```python
from build123d import *

# Parameters (mm, degrees)
SKETCH1_R           = 0.375
SKETCH1_R_2         = 0.6
BOSS_EXTRUDE1_DEPTH = 1.25
BOSS_EXTRUDE2_DEPTH = 2.4
BOSS_EXTRUDE3_DEPTH = 4


with BuildPart() as part:
    # Sketch1 → Boss-Extrude1 (new body)
    # profile 1 of 7: a face of its own
    with BuildSketch(Plane(origin=(0, 0, 0), x_dir=(1, 0, 0), z_dir=(0, 1, 0))):
        with BuildLine():
            Line((18.75, 18.75), (13.75, 18.75))
            ThreePointArc((13.75, 18.75), (12.5, 17.5), (11.25, 18.75))
            Line((11.25, 18.75), (-18.75, 18.75))
            Line((-18.75, 18.75), (-18.75, -18.75))
            Line((-18.75, -18.75), (11.25, -18.75))
            ThreePointArc((11.25, -18.75), (12.5, -17.5), (13.75, -18.75))
            Line((13.75, -18.75), (18.75, -18.75))
            Line((18.75, -18.75), (18.75, 18.75))
        make_face()
        with Locations((-18, -18)):
            Circle(SKETCH1_R, mode=Mode.SUBTRACT)
        with BuildLine():
            ThreePointArc((-5.25, 17), (-4.542893219, 16.707106781), (-4.25, 16))
            Line((-4.25, 16), (-4.25, 15.75))
            ThreePointArc((-4.25, 15.75), (-3.957106781, 15.042893219), (-3.25, 14.75))
            Line((-3.25, 14.75), (3.25, 14.75))
            ThreePointArc((3.25, 14.75), (3.957106781, 15.042893219), (4.25, 15.75))
            Line((4.25, 15.75), (4.25, 16))
            ThreePointArc((4.25, 16), (4.542893219, 16.707106781), (5.25, 17))
            Line((5.25, 17), (12, 17))
            ThreePointArc((12, 17), (15.535533906, 15.535533906), (17, 12))
            Line((17, 12), (17, -12))
            ThreePointArc((17, -12), (15.535533906, -15.535533906), (12, -17))
            Line((12, -17), (-12, -17))
            ThreePointArc((-12, -17), (-15.535533906, -15.535533906), (-17, -12))
            Line((-17, -12), (-17, 12))
            ThreePointArc((-17, 12), (-15.535533906, 15.535533906), (-12, 17))
            Line((-12, 17), (-5.25, 17))
        make_face(mode=Mode.SUBTRACT)
        with Locations((16.95, -16.95)):
            Circle(SKETCH1_R_2, mode=Mode.SUBTRACT)
        with Locations((-18, 18)):
            Circle(SKETCH1_R, mode=Mode.SUBTRACT)
        Polygon((16.75, 18.25), (18.25, 18.25), (18.25, 16.75), align=None, mode=Mode.SUBTRACT)
    # profile 2 of 7: a face of its own
    with BuildSketch(Plane(origin=(0, 0, 0), x_dir=(1, 0, 0), z_dir=(0, 1, 0))):
        with BuildLine():
            Line((-4.25, 15.75), (-4.25, 16))
            ThreePointArc((-4.25, 16), (-4.542893219, 16.707106781), (-5.25, 17))
            Line((-5.25, 17), (-12, 17))
            ThreePointArc((-12, 17), (-15.535533906, 15.535533906), (-17, 12))
            Line((-17, 12), (-17, -12))
            ThreePointArc((-17, -12), (-15.535533906, -15.535533906), (-12, -17))
            Line((-12, -17), (12, -17))
            ThreePointArc((12, -17), (15.535533906, -15.535533906), (17, -12))
            Line((17, -12), (17, 12))
            ThreePointArc((17, 12), (15.535533906, 15.535533906), (12, 17))
            Line((12, 17), (5.25, 17))
            ThreePointArc((5.25, 17), (4.542893219, 16.707106781), (4.25, 16))
            Line((4.25, 16), (4.25, 15.75))
            ThreePointArc((4.25, 15.75), (3.957106781, 15.042893219), (3.25, 14.75))
            Line((3.25, 14.75), (12.25, 14.75))
            ThreePointArc((12.25, 14.75), (14.017766953, 14.017766953), (14.75, 12.25))
            Line((14.75, 12.25), (14.75, -12.25))
            ThreePointArc((14.75, -12.25), (14.017766953, -14.017766953), (12.25, -14.75))
            Line((12.25, -14.75), (-12.25, -14.75))
            ThreePointArc((-12.25, -14.75), (-14.017766953, -14.017766953), (-14.75, -12.25))
            Line((-14.75, -12.25), (-14.75, 12.25))
            ThreePointArc((-14.75, 12.25), (-14.017766953, 14.017766953), (-12.25, 14.75))
            Line((-12.25, 14.75), (-3.25, 14.75))
            ThreePointArc((-3.25, 14.75), (-3.957106781, 15.042893219), (-4.25, 15.75))
        make_face()
    # profile 3 of 7: a face of its own
    with BuildSketch(Plane(origin=(0, 0, 0), x_dir=(1, 0, 0), z_dir=(0, 1, 0))):
        with BuildLine():
            Line((12.25, 14.75), (-12.25, 14.75))
            ThreePointArc((-12.25, 14.75), (-14.017766953, 14.017766953), (-14.75, 12.25))
            Line((-14.75, 12.25), (-14.75, -12.25))
            ThreePointArc((-14.75, -12.25), (-14.017766953, -14.017766953), (-12.25, -14.75))
            Line((-12.25, -14.75), (12.25, -14.75))
            ThreePointArc((12.25, -14.75), (14.017766953, -14.017766953), (14.75, -12.25))
            Line((14.75, -12.25), (14.75, 12.25))
            ThreePointArc((14.75, 12.25), (14.017766953, 14.017766953), (12.25, 14.75))
        make_face()
    # profile 4 of 7: a face of its own
    with BuildSketch(Plane(origin=(0, 0, 0), x_dir=(1, 0, 0), z_dir=(0, 1, 0))):
        with Locations((-18, -18)):
            Circle(SKETCH1_R)
    # profile 5 of 7: a face of its own
    with BuildSketch(Plane(origin=(0, 0, 0), x_dir=(1, 0, 0), z_dir=(0, 1, 0))):
        with Locations((16.95, -16.95)):
            Circle(SKETCH1_R_2)
    # profile 6 of 7: a face of its own
    with BuildSketch(Plane(origin=(0, 0, 0), x_dir=(1, 0, 0), z_dir=(0, 1, 0))):
        Polygon((18.25, 18.25), (16.75, 18.25), (18.25, 16.75), align=None)
    # profile 7 of 7: a face of its own
    with BuildSketch(Plane(origin=(0, 0, 0), x_dir=(1, 0, 0), z_dir=(0, 1, 0))):
        with Locations((-18, 18)):
            Circle(SKETCH1_R)
    extrude(amount=BOSS_EXTRUDE1_DEPTH)

    # Sketch1_3 → Boss-Extrude2 (add)
    with BuildSketch(Plane(origin=(0, 0, 0), x_dir=(1, 0, 0), z_dir=(0, 1, 0))):
        with BuildLine():
            Line((-4.25, 15.75), (-4.25, 16))
            ThreePointArc((-4.25, 16), (-4.542893219, 16.707106781), (-5.25, 17))
            Line((-5.25, 17), (-12, 17))
            ThreePointArc((-12, 17), (-15.535533906, 15.535533906), (-17, 12))
            Line((-17, 12), (-17, -12))
            ThreePointArc((-17, -12), (-15.535533906, -15.535533906), (-12, -17))
            Line((-12, -17), (12, -17))
            ThreePointArc((12, -17), (15.535533906, -15.535533906), (17, -12))
            Line((17, -12), (17, 12))
            ThreePointArc((17, 12), (15.535533906, 15.535533906), (12, 17))
            Line((12, 17), (5.25, 17))
            ThreePointArc((5.25, 17), (4.542893219, 16.707106781), (4.25, 16))
            Line((4.25, 16), (4.25, 15.75))
            ThreePointArc((4.25, 15.75), (3.957106781, 15.042893219), (3.25, 14.75))
            Line((3.25, 14.75), (12.25, 14.75))
            ThreePointArc((12.25, 14.75), (14.017766953, 14.017766953), (14.75, 12.25))
            Line((14.75, 12.25), (14.75, -12.25))
            ThreePointArc((14.75, -12.25), (14.017766953, -14.017766953), (12.25, -14.75))
            Line((12.25, -14.75), (-12.25, -14.75))
            ThreePointArc((-12.25, -14.75), (-14.017766953, -14.017766953), (-14.75, -12.25))
            Line((-14.75, -12.25), (-14.75, 12.25))
            ThreePointArc((-14.75, 12.25), (-14.017766953, 14.017766953), (-12.25, 14.75))
            Line((-12.25, 14.75), (-3.25, 14.75))
            ThreePointArc((-3.25, 14.75), (-3.957106781, 15.042893219), (-4.25, 15.75))
        make_face()
        with BuildLine():
            Line((12.25, 14.75), (-12.25, 14.75))
            ThreePointArc((-12.25, 14.75), (-14.017766953, 14.017766953), (-14.75, 12.25))
            Line((-14.75, 12.25), (-14.75, -12.25))
            ThreePointArc((-14.75, -12.25), (-14.017766953, -14.017766953), (-12.25, -14.75))
            Line((-12.25, -14.75), (12.25, -14.75))
            ThreePointArc((12.25, -14.75), (14.017766953, -14.017766953), (14.75, -12.25))
            Line((14.75, -12.25), (14.75, 12.25))
            ThreePointArc((14.75, 12.25), (14.017766953, 14.017766953), (12.25, 14.75))
        make_face()
    extrude(amount=BOSS_EXTRUDE2_DEPTH)

    # Sketch1_4 → Boss-Extrude3 (add)
    with BuildSketch(Plane(origin=(0, 0, 0), x_dir=(1, 0, 0), z_dir=(0, 1, 0))):
        with BuildLine():
            Line((12.25, 14.75), (-12.25, 14.75))
            ThreePointArc((-12.25, 14.75), (-14.017766953, 14.017766953), (-14.75, 12.25))
            Line((-14.75, 12.25), (-14.75, -12.25))
            ThreePointArc((-14.75, -12.25), (-14.017766953, -14.017766953), (-12.25, -14.75))
            Line((-12.25, -14.75), (12.25, -14.75))
            ThreePointArc((12.25, -14.75), (14.017766953, -14.017766953), (14.75, -12.25))
            Line((14.75, -12.25), (14.75, 12.25))
            ThreePointArc((14.75, 12.25), (14.017766953, 14.017766953), (12.25, 14.75))
        make_face()
    extrude(amount=BOSS_EXTRUDE3_DEPTH)


solid = part.part
```
The listing builds one solid part. Answer for the finished solid, in the listing's coordinates (mm). A direction names the side the tool comes from. Round coordinates to 2 decimals unless told otherwise and drop trailing zeros. Loops run counter-clockwise (first coordinate to the right, second up) from the corner with the lowest first, then second, coordinate; pieces in that order, holes last.
Q1. Given pin 1 Ø0.6 at (x, y) = (2, 1.5) entering from +Z; pin 2 Ø1.4 at (x, y) = (0, 2) entering from -Z; pin 3 Ø1.3 at (y, z) = (3, 3.5) entering from -X; pin 4 Ø0.8 at (y, z) = (3.5, 4) entering from +X, each flat-ended and moving along its own axis, determine where each tip first touches the part or whether it passes through.
Q2. For a pull along X with two mould halves and no side action, classify faces 5 (the face through (-14.037, 3.189, 13.998)), 6 (the face through (16, 1, 18.75)), 7 (the face through (-3.949, 1.817, -15.035)), 8 (the face through (14.75, 3, 0)) as released by +X, released by -X, zero draft, split by the parting line, or undercut.
Q3. Section B-B, the plane y = 3.4 is taken. Determine the outline of the cut face in (x, z), then the cut area to 3 significant figures.
Q4. Section A-A, the plane x = -6 is taken. Determine the outline of the cut face in (y, z), then the cut area to 3 significant figures.
Q5. Which of the six approach directions +Z, -Z, +X, -X, +Y, -Y give full straight-line access (tool end or side, diameter ignored) to faces 1 (the face through (9, 2, -17)), 2 (the face through (13.998, 3.189, 14.037)), 3 (the face through (0, 2.4, 15)), 4 (the face through (-4.535, 1.817, -16.699))?
Q6. Section D-D, the plane x = 1 is taken. Determine the outline of the cut face in (y, z), then the cut area to 3 significant figures.
Q7. Find the intervals of material crossed by line 1 (Z direction, x = -2, y = 3.55); line 2 (Y direction, x = -2, z = 17.5); line 3 (X direction, y = 1.75, z = 9), in increasing order.
Q8. Section C-C, the plane z = 10.5 is taken. Determine the outline of the cut face in (x, y), then the cut area to 3 significant figures.
Completed:
1. pin 1: stops at z = 18.75
1. pin 2: stops at z = -14.75
1. pin 3: stops at x = -17
1. pin 4: stops at x = 14.75
2. face 5: released by -X
2. face 6: zero draft
2. face 7: undercut
2. face 8: released by +X
3. outline: (-14.75, -12.25) arc R2.5 ccw to (-12.25, -14.75) - (12.25, -14.75) arc R2.5 ccw to (14.75, -12.25) - (14.75, 12.25) arc R2.5 ccw to (12.25, 14.75) - (-12.25, 14.75) arc R2.5 ccw to (-14.75, 12.25) - close
3. area: 865 mm2
4. outline: (0, -18.75) - (1.25, -18.75) - (1.25, -17) - (2.4, -17) - (2.4, -14.75) - (4, -14.75) - (4, 14.75) - (2.4, 14.75) - (2.4, 17) - (1.25, 17) - (1.25, 18.75) - (0, 18.75) - close
4. area: 133 mm2
5. face 1: -Z, +X, -X, +Y
5. face 2: +Z, +X, +Y
5. face 3: +Y
5. face 4: -Z, +Y
6. outline: (0, -18.75) - (1.25, -18.75) - (1.25, -14.75) - (4, -14.75) - (4, 14.75) - (2.4, 14.75) - (2.4, 17) - (1.25, 17) - (1.25, 18.75) - (0, 18.75) - close
6. area: 131 mm2
7. line 1: z = -14.75 to 14.75
7. line 2: y = 0 to 1.25
7. line 3: x = -17 to 17
8. outline: (-18.75, 0) - (18.75, 0) - (18.75, 1.25) - (17, 1.25) - (17, 2.4) - (14.75, 2.4) - (14.75, 4) - (-14.75, 4) - (-14.75, 2.4) - (-17, 2.4) - (-17, 1.25) - (-18.75, 1.25) - close
8. area: 133 mm2
